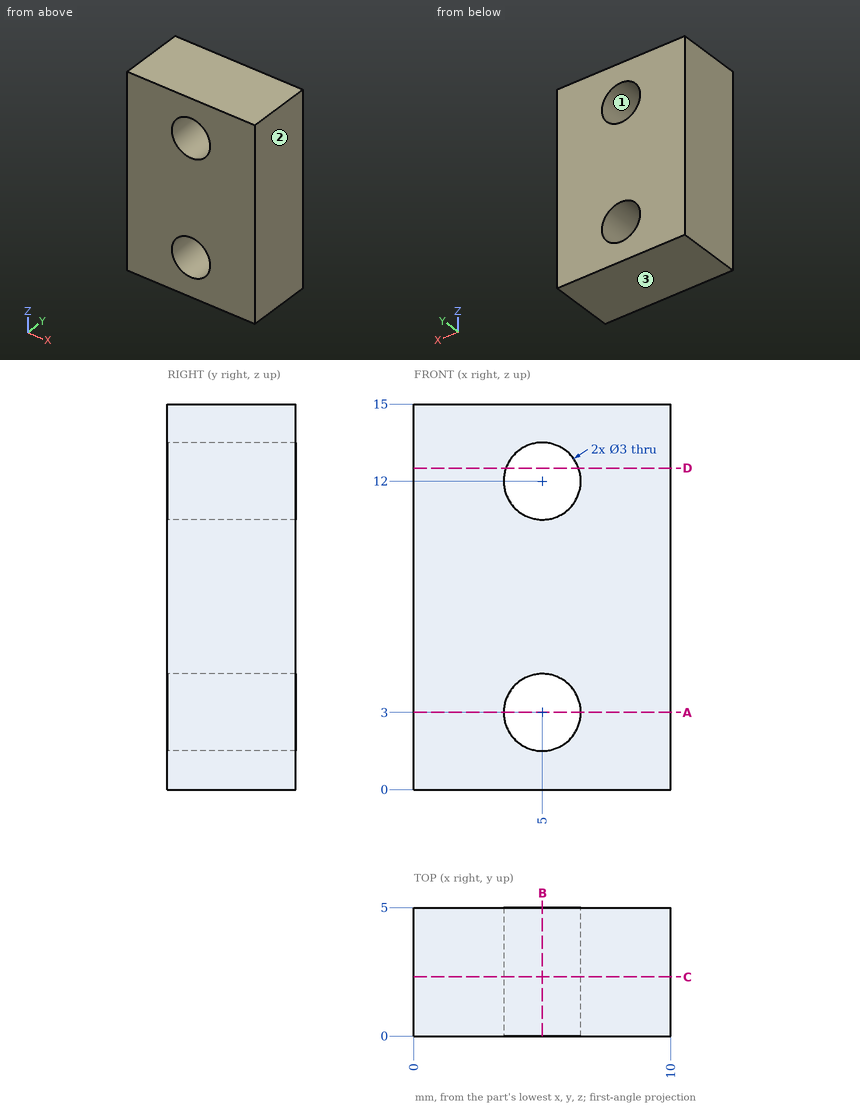
Check sheet for the drawn part. Datum: minimum x, y, z corner. Units: mm. Round coordinates to 2 decimals unless told otherwise and drop trailing zeros. Write each loop counter-clockwise with the first axis right and the second up, starting at its lowest first coordinate (ties: lowest second). Pieces come first, ordered by that corner, then holes. Notation, with made-up numbers: (-26, 57) -> (14, 57) arc R13 ccw to (14, 72) -> close; hole circle Ø10 at (43.5, 51). An arc over 180 degrees is marked (long way). One line per item, written item: value. Start each with the question number.
(1) Go/stop test with a flat-tipped pin: pin 1 Ø4 at (x, z) = (4, 13.5) entering from -Y. Record where the tip stops, or that it passes through.
(2) Draft check along Z on the marked faces 1, 2 and 3. Enter one of: +Z half, -Z half, draft (parallel to the pull), parting line (faces both ways), or undercut.
(3) Cross-section at A-A, the plane z = 3. Record the cut outline in (x, y), and give its area (3 significant figures).
(4) Scan lines: line 1 (Z direction, x = 5, y = 4.05); line 2 (Z direction, x = 4.5, y = 0.75); line 3 (X direction, y = 4.45, z = 12.25). Record each from-to range of solid material in increasing order. Write a range as [from, to].
(5) Cross-section at D-D, the plane z = 12.5. Record the cut outline in (x, y).
(6) Cross-section at C-C, the plane y = 2.3. Record the cut outline in (x, z).
(7) Cross-section at B-B, the plane x = 5. Record the cut outline in (y, z).
Answer:
1. pin 1: y = 0
2. face 1: undercut
2. face 2: draft
2. face 3: -Z half
3. outline: (0, 0) -> (3.5, 0) -> (3.5, 5) -> (0, 5) -> close; (6.5, 0) -> (10, 0) -> (10, 5) -> (6.5, 5) -> close
3. area: 35.0 mm²
4. line 1: [0, 1.5], [4.5, 10.5], [13.5, 15]
4. line 2: [0, 1.59], [4.41, 10.59], [13.41, 15]
4. line 3: [0, 3.52], [6.48, 10]
5. outline: (0, 0) -> (3.59, 0) -> (3.59, 5) -> (0, 5) -> close; (6.41, 0) -> (10, 0) -> (10, 5) -> (6.41, 5) -> close
6. outline: (0, 0) -> (10, 0) -> (10, 15) -> (0, 15) -> close; hole circle Ø3 at (5, 3); hole circle Ø3 at (5, 12)
7. outline: (0, 0) -> (5, 0) -> (5, 1.5) -> (0, 1.5) -> close; (0, 4.5) -> (5, 4.5) -> (5, 10.5) -> (0, 10.5) -> close; (0, 13.5) -> (5, 13.5) -> (5, 15) -> (0, 15) -> close
